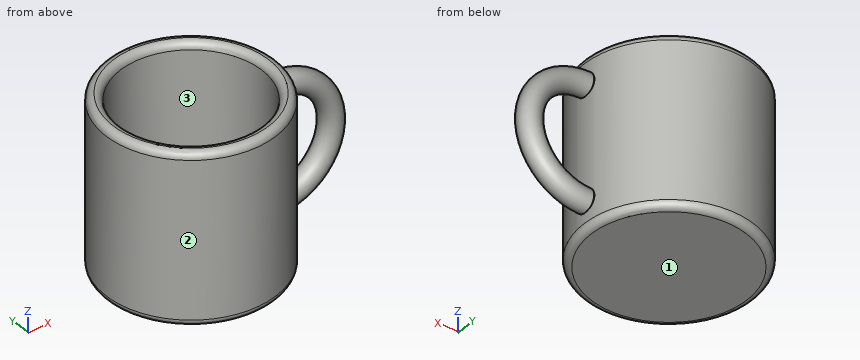
from build123d import *
from build123d import SkipClean  # not in build123d's __all__

# Parameters (mm, degrees)
F0_W      = 19.05
F0_H      = 38.1
F2_R      = 15.875
F3_DEPTH  = 34.925
F6_R      = 1.58749
F7_R      = 1.5875
F8_R      = 2.54
F10_R     = 2.54
F11_R     = 2.54
F12_DEPTH = 3.175


# Not quite as in the source:
# - a fillet or chamfer is up to 0.001 mm smaller than in the source, because OpenCascade refuses the exact size


with BuildPart() as f1:
    # F0 (on Front) → F1 (revolve)
    with BuildSketch(Plane.XZ):
        with Locations((9.525, 19.05)):
            Rectangle(F0_W, F0_H)
    revolve(axis=Axis((0, 0, 19.05), (0, 0, 1)))

    # F2 (on face) → F3 (cut)
    with BuildSketch(Plane.XY.offset(38.1)):
        Circle(F2_R)
    extrude(amount=-F3_DEPTH, mode=Mode.SUBTRACT)

    # F6 (radius 1.5875 in the source; OpenCascade refuses exactly that, so slightly less here)
    f6_edges = [f1.edges().sort_by_distance(p)[0] for p in [
        (-19.05, 0, 38.1),
        (-15.875, 0, 38.1),
    ]]
    fillet(f6_edges, radius=F6_R)

    # F7
    f7_edges = [f1.edges().sort_by_distance(p)[0] for p in [
        (-19.05, 0, 0),
    ]]
    fillet(f7_edges, radius=F7_R)

    # F9: sweep along a path in F5
    with BuildLine(Plane.XZ) as f9_path:
        ThreePointArc((19.05, 6.35), (31.75, 19.05), (19.05, 31.75))
    # F8 (on offset) → F9 (sweep)
    with BuildSketch(Plane.YZ.offset(19.05)):
        with Locations((0, 31.75)):
            Circle(F8_R)
    sweep(path=f9_path.line)

    # F10 (on face) + F11 (on face) → F12 (join, through all)
    with BuildSketch(Plane(origin=(19.05, 0, 0), x_dir=(0, -1, 0), z_dir=(-1, 0, 0))):
        with Locations((0, 31.75)):
            Circle(F10_R)
    with BuildSketch(Plane(origin=(19.05, 0, 0), x_dir=(0, -1, 0), z_dir=(-1, 0, 0))):
        with Locations((0, 6.35)):
            Circle(F11_R)
    with SkipClean():  # cleaning this boolean's faces spoils the solid; the shape is the same uncleaned
        extrude(amount=F12_DEPTH)


solid = f1.part
Geometry check sheet. Reference: the model listing, model coordinates, mm. Face numbers are marked on the shaded views. Give positions to 0.01 mm unless a question says otherwise; leave off trailing zeros. Write each question's results on one line, items separated by ' | '.
1) Release check for a two-part mould opening along Y. For the marked faces 1, 2 and 3 record: +Y half, -Y half, draft (parallel to the pull), parting line (faces both ways), or undercut.
Answers follow:
face 1: draft | face 2: parting line | face 3: undercut
2) Gauge pin test, flat ends, axial feed: pin 1 (10 mm diameter, centred on x = -5.5, y = 7, fed in from +Z) (3 decimals); pin 2 (1 mm diameter, centred on x = 20, z = 31, fed in from +Y); pin 3 (6 mm diameter, centred on x = 2, z = 12.5, fed in from -Y). Record the tip position at first contact, or that the pin passes through.
Answers follow:
pin 1: z = 3.175 | pin 2: y = 2.53 | pin 3: y = -19.05
3) Thickness scan on line 1 (Y direction, x = 0, z = 29) (3 decimals); line 2 (Z direction, x = -5, y = -1) (3 decimals); line 3 (X direction, y = 0.5, z = 24). Record the ranges inside material, lowest first.
Answers follow:
line 1: -19.05 to -15.875, 15.875 to 19.05 | line 2: 0 to 3.175 | line 3: -19.04 to -15.87, 15.87 to 19.04, 27.98 to 33.41
4) Section check B-B, the plane z = 25.5. Count the separate pieces of the cut face and the enclosed holes in it, plus the area to 3 significant figures.
Answers follow:
separate pieces: 2 | enclosed holes: 1 | area: 372 mm2
